```python
from build123d import *

# Parameters (mm, degrees)
SKETCH2_R           = 5.08
BOSS_EXTRUDE2_DEPTH = 41.91
SKETCH3_W           = 8.89
SKETCH3_H           = 6.35
SKETCH6_R           = 2.54
CUT_EXTRUDE1_DEPTH  = 17.78
SKETCH7_R           = 2.54
CUT_EXTRUDE2_DEPTH  = 19.05


with BuildPart() as part:
    # Sketch2 → Boss-Extrude2 (new body)
    with BuildSketch(Plane(origin=(0, 0, 0), x_dir=(-1, 0, 0), z_dir=(0, 1, 0))):
        with Locations(Location((0, 0, 0), (0, 0, 90))):
            Circle(SKETCH2_R)
    extrude(amount=BOSS_EXTRUDE2_DEPTH)

    # Sketch3 → Revolve1 (revolve)
    with BuildSketch(Plane.XY, mode=Mode.PRIVATE) as revolve1_sk:
        with Locations((-4.445, 10.795)):
            Rectangle(SKETCH3_W, SKETCH3_H)
    revolve(revolve1_sk.sketch.rotate(Axis((0, 0, 0), (0, 1, 0)), 270), axis=Axis((0, 0, 0), (0, 1, 0)))

    # Sketch4 → Revolve2 (revolve)
    with BuildSketch(Plane(origin=(0, 41.91, 0), x_dir=(1, 0, 0), z_dir=(0, 1, 0)), mode=Mode.PRIVATE) as revolve2_sk:
        with BuildLine():
            Line((0, 5.08), (-84.328, 5.08))
            Line((-84.328, 5.08), (-84.328, 0))
            Line((-84.328, 0), (5.08, 0))
            ThreePointArc((5.08, 0), (3.592102448, 3.592102448), (0, 5.08))
        make_face()
    revolve(revolve2_sk.sketch.rotate(Axis((-84.328, 41.91, 0), (1, 0, 0)), 180), axis=Axis((-84.328, 41.91, 0), (1, 0, 0)))

    # Sketch5 → Revolve3 (revolve)
    with BuildSketch(Plane.ZY.offset(84.328), mode=Mode.PRIVATE) as revolve3_sk:
        with BuildLine():
            Line((0, 46.99), (0, 24.13))
            Line((0, 24.13), (-5.08, 24.13))
            Line((-5.08, 24.13), (-5.08, 41.91))
            ThreePointArc((-5.08, 41.91), (-3.592102448, 45.502102448), (0, 46.99))
        make_face()
    revolve(revolve3_sk.sketch.rotate(Axis((-84.328, 46.99, 0), (0, -1, 0)), 180), axis=Axis((-84.328, 46.99, 0), (0, -1, 0)))

    # Sketch6 → Cut-Extrude1 (cut)
    with BuildSketch(Plane.XZ.offset(-24.13)):
        with Locations(Location((-84.328, 0, 0), (0, 0, 270))):
            Circle(SKETCH6_R)
    extrude(amount=-CUT_EXTRUDE1_DEPTH, mode=Mode.SUBTRACT)

    # Sketch7 → Cut-Extrude2 (cut)
    with BuildSketch(Plane.XZ):
        with Locations(Location((0, 0, 0), (0, 0, 270))):
            Circle(SKETCH7_R)
    extrude(amount=-CUT_EXTRUDE2_DEPTH, mode=Mode.SUBTRACT)


solid = part.part
```
The model under review builds one solid part; all positions refer to its coordinate system, in mm. A direction names the side the tool comes from. Give positions to 0.01 mm unless a question says otherwise; leave off trailing zeros. Write each loop counter-clockwise with the first axis right and the second up, starting at its lowest first coordinate (ties: lowest second). Pieces come first, ordered by that corner, then holes. Notation, with made-up numbers: (-14.75, -3) -> (-5.75, -3) arc R13 ccw to (-5.75, 8) -> close; hole circle Ø5 at (87, -20.75). An arc over 180 degrees is marked (long way). Answer in a Markdown table with one row per item.
1) For L1, parallel to X at y = 30.25, z = 0; L2, parallel to X at y = 8, z = 0; L3, parallel to X at y = 6.5, z = 0, list the stretches that pass through material, from the lowest coordinate up. Write a range as [from, to].
Worked answers:
| item | result |
|---|---|
| L1 | [-89.41, -86.87], [-81.79, -79.25], [-5.08, 5.08] |
| L2 | [-8.89, -2.54], [2.54, 8.89] |
| L3 | [-5.08, -2.54], [2.54, 5.08] |
2) Add section D-D on y = 21. State the section outline as (x, z) points.
Worked answers:
| item | result |
|---|---|
| outline | circle Ø10.16 at (0, 0) |
3) Tool access review of faces 5 (the cylindrical face through (2.52, 9.39, 0.33)), 6 (the flat face through (-87, 24.13, -1)), 7 (the flat face through (4, 13.97, -4)): name each direction out of +Z, -Z, +X, -X, +Y, -Y from which nothing blocks a thin tool from reaching the whole face with its end or side.
Worked answers:
| item | result |
|---|---|
| face 5 | -Y |
| face 6 | +Z, -Z, -X, -Y |
| face 7 | none |
4) Add section A-A on z = 0. State the section outline as (x, y) points.
Worked answers:
| item | result |
|---|---|
| outline | (-89.41, 24.13) -> (-86.87, 24.13) -> (-86.87, 41.91) -> (-81.79, 41.91) -> (-81.79, 24.13) -> (-79.25, 24.13) -> (-79.25, 36.83) -> (-5.08, 36.83) -> (-5.08, 13.97) -> (-8.89, 13.97) -> (-8.89, 7.62) -> (-5.08, 7.62) -> (-5.08, 0) -> (-2.54, 0) -> (-2.54, 19.05) -> (2.54, 19.05) -> (2.54, 0) -> (5.08, 0) -> (5.08, 7.62) -> (8.89, 7.62) -> (8.89, 13.97) -> (5.08, 13.97) -> (5.08, 41.91) arc R5.08 ccw to (0, 46.99) -> (-84.33, 46.99) arc R5.08 ccw to (-89.41, 41.91) -> close |
5) Add section B-B on y = 16. State the section outline as (x, z) points, plus the area to 3 significant figures.
Worked answers:
| item | result |
|---|---|
| outline | circle Ø10.16 at (0, 0); hole circle Ø5.08 at (0, 0) |
| area | 60.8 mm² |
6) Add section C-C on x = -64. State the section outline as (y, z) points, plus the area to 3 significant figures.
Worked answers:
| item | result |
|---|---|
| outline | circle Ø10.16 at (41.91, 0) |
| area | 81.1 mm² |
7) Mouldability with a two-part tool opening along X and no side actions: class faces 1 (the cylindrical face through (-86.808, 32.896, 0.551)), 2 (the cylindrical face through (5.037, 3.757, -0.661)), 3 (the cylindrical face through (-89.365, 33.144, -0.661)), 4 (the flat face through (-2, 0, 2)) as +X half, -X half, draft (parallel to the pull), parting line (faces both ways), or undercut.
Worked answers:
| item | result |
|---|---|
| face 1 | undercut |
| face 2 | parting line |
| face 3 | undercut |
| face 4 | draft |
8) Clearance check with flat-ended pins moving along their axes: P1, Ø1.5, axis at x = 0, z = 0, coming from the -Y side; P2, Ø5.5, axis at x = 0.5, z = 3.5, coming from the +Y side; P3, Ø1, axis at y = 5, z = 4.5, coming from the -X side. State where each tip first meets the part, or that it passes through.
Worked answers:
| item | result |
|---|---|
| P1 | y = 19.05 |
| P2 | y = 46.93 |
| P3 | x = -3.13 |
